Autodesk Inventor part; units mm, degrees
ref_plane "YZ Plane" through (0, 0, 0) normal (1, 0, 0) x (0, 1, 0)
ref_plane "XZ Plane" through (0, 0, 0) normal (0, 1, 0) x (-1, 0, 0)
ref_plane "XY Plane" through (0, 0, 0) normal (0, 0, 1) x (1, 0, 0)
sketch "Sketch1" plane through (0, 0, 0) normal (0, 0, 1) x (1, 0, 0)
  line L0 (-24.9, 0) -> (-25.4, 0.5)
  line L1 (-16.6687, 0) -> (-24.9, 0)
  line L2 (-16.6687, 1.5875) -> (-16.6687, 0)
  line L3 (-14.3002, 1.5875) -> (-16.6687, 1.5875)
  line L4 (-14.3002, 3) -> (-14.3002, 1.5875)
  line L5 (-24.9, 3) -> (-14.3002, 3)
  line L6 (-25.4, 2.5) -> (-24.9, 3)
  line L7 (-25.4, 0.5) -> (-25.4, 2.5)
  line L8 (0, 0) -> (0, 6.8981)
  dimension "d0" = 50.8
  dimension "d1" = 28.6004
  dimension "d2" = 3
  dimension "d3" = 1.5875
  dimension "d4" = 2.3685
  dimension "d5" = 0.5
  dimension "d6" = 0.5
  dimension "d7" = 0.5
  dimension "d9" = 0.5
revolve "Revolution1" add sketch "Sketch1" angle 360 about axis through (0, 0, 0) along (0, 1, 0)
equation "\"d6\" = d5"
equation "\"d9\" = d7"
properties part number "VersaRoller Flange (WCP-0444)" material "Aluminum 6061"
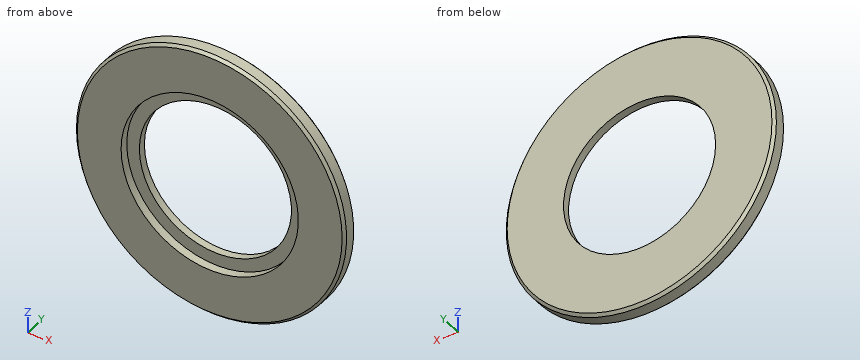
Work out the finished part from the listing and answer in its coordinate system (mm). Round coordinates to 2 decimals unless told otherwise and drop trailing zeros. Order: outer loops, then holes, each group sorted by start corner. A loop starts at its lowest first (then second) coordinate and runs counter-clockwise, first axis right, second up. Notation, with made-up numbers: M 28,29 L 73,29 A36 cw 73,65 Z; hole C -23,61.5 d4. An arc over 180 degrees is marked long. One line per item, written item: value.
Q1. Flat-ended cylindrical pins translate along their axes: pin 1 (23 mm diameter, centred on x = 0, z = 0, fed in from +Y); pin 2 (1.5 mm diameter, centred on x = 0, y = 0.5, fed in from -Z). Find the tip coordinate at first contact, or state that the pin passes through.
Derived:
pin 1: through
pin 2: z = -25.4
Q2. Straight lines are drawn through the part: line 1 (Z direction, x = 0, y = 1.1); line 2 (X direction, y = 2.3, z = 12); line 3 (Z direction, x = -12, y = 0.8). For each, find the intervals that lie inside material, in ascending order.
Derived:
line 1: -25.4 to -16.67, 16.67 to 25.4
line 2: -22.39 to -7.78, 7.78 to 22.39
line 3: -22.39 to -11.57, 11.57 to 22.39
Q3. Find section B-B on x = 0. Write down the section's boundary in (y, z), then the cut area to 3 significant figures.
Derived:
outline: M 0,-24.9 L 0.5,-25.4 L 2.5,-25.4 L 3,-24.9 L 3,-14.3 L 1.59,-14.3 L 1.59,-16.67 L 0,-16.67 Z; M 0,16.67 L 1.59,16.67 L 1.59,14.3 L 3,14.3 L 3,24.9 L 2.5,25.4 L 0.5,25.4 L 0,24.9 Z
area: 58.6 mm²
Q4. Find section A-A on z = 0. Write down the section's boundary in (x, y), then the cut area to 3 significant figures.
Derived:
outline: M -25.4,0.5 L -24.9,0 L -16.67,0 L -16.67,1.59 L -14.3,1.59 L -14.3,3 L -24.9,3 L -25.4,2.5 Z; M 14.3,1.59 L 16.67,1.59 L 16.67,0 L 24.9,0 L 25.4,0.5 L 25.4,2.5 L 24.9,3 L 14.3,3 Z
area: 58.6 mm²
